Source: CAD feature listing. Evaluate the final solid. Frame: model axes, mm. A direction names the side the tool comes from. Coordinates: 2 decimals unless noted, no trailing zeros. Order: outer loops, then holes, each group sorted by start corner. A loop starts at its lowest first (then second) coordinate and runs counter-clockwise, first axis right, second up. Notation, with made-up numbers: (35, 88.25) - (56, 88.25) arc R18 ccw to (56, 106.25) - close; hole circle Ø4 at (23.25, 2). An arc over 180 degrees is marked (long way). One line per question, with ' | ' between items. Start each with the question number.
(1) Section B-B (y = 30.5). Return the cut outline in (x, z), then the cut area to 3 significant figures.
(2) Section C-C (y = 4). Return the cut outline in (x, z), then the cut area to 3 significant figures.
(3) Contact query for flat-ended pins moving along their axis: P1, Ø3, axis at x = 28, y = 22.44, coming from the +Z side; P2, Ø2, axis at x = 89.5, z = 0.5, coming from the +Y side. Output: stop coordinate, or through.
(4) Access query for faces 1 (the cylindrical face through (-9.54, 20, 0.03)), 2 (the flat face through (-42, 22, 0)). Directions: +Z, -Z, +X, -X, +Y, -Y. A direction counts if a zero-diameter tool reaches every point of the face in a straight line with its end or side. Return the directions, or none.
(5) Line query: line 1 along X through (y, z) = (14.5, 0.45); line 2 along Y through (x, z) = (28, -0.75); line 3 along X through (y, z) = (2, -1.7). Output: solid intervals per line, ascending.
(6) Draft query along Y for faces 3 (the flat face through (83, 12.443, 0)), 4 (the flat face through (27, 8, 2)), 5 (the cylindrical face through (103.154, 20.225, 0.028)), 6 (the cylindrical face through (67.31, 21.49, 0.03)). Return one class per face: +Y half, -Y half, draft (parallel to the pull), parting line (faces both ways), or undercut.
(7) Section D-D (z = 0.8). Count the separate pieces of the cut face and the enclosed holes in it, then the cut area to 3 significant figures.
(8) Section A-A (x = -46). Return the cut outline in (y, z).
from build123d import *

# Parameters (mm, degrees)
SKETCH1_W           = 156
SKETCH1_H           = 20
SKETCH1_W_2         = 8
BOSS_EXTRUDE1_DEPTH = 2
SKETCH2_R           = 2.5
CUT_EXTRUDE1_DEPTH  = 111.92580296
LPATTERN1_COUNT     = 5
LPATTERN1_PITCH     = 37
SKETCH3_R           = 3
CUT_EXTRUDE2_DEPTH  = 111.92580296


with BuildPart() as part:
    # Sketch1 → Boss-Extrude1 (new, symmetric)
    with BuildSketch(Plane.XY):
        with Locations((28, 2.442776735)):
            Rectangle(SKETCH1_W, SKETCH1_H)
        with Locations((102, 22.442776735)):
            Rectangle(SKETCH1_W_2, SKETCH1_H)
        with Locations((65, 22.442776735)):
            Rectangle(SKETCH1_W_2, SKETCH1_H)
        with Locations((28, 22.442776735)):
            Rectangle(SKETCH1_W_2, SKETCH1_H)
        with Locations((-9, 22.442776735)):
            Rectangle(SKETCH1_W_2, SKETCH1_H)
        with Locations((-46, 22.442776735)):
            Rectangle(SKETCH1_W_2, SKETCH1_H)
    extrude(amount=BOSS_EXTRUDE1_DEPTH, both=True)

    # Sketch2 → Cut-Extrude1 (cut, through all)
    with BuildSketch(Plane.XY.offset(2)):
        with Locations((-46, 22.442776735)):
            Circle(SKETCH2_R)
    cut_extrude1 = extrude(amount=-CUT_EXTRUDE1_DEPTH, mode=Mode.SUBTRACT)

    # LPattern1: Cut-Extrude1 ×5
    with Locations(*[(i * LPATTERN1_PITCH, 0, 0) for i in range(1, LPATTERN1_COUNT)]):
        add(cut_extrude1, mode=Mode.SUBTRACT)

    # Sketch3 → Cut-Extrude2 (cut, through all)
    with BuildSketch(Plane.XY.offset(2)):
        with Locations((28, 2.442776735)):
            Circle(SKETCH3_R)
        with Locations((96, 2.442776735)):
            Circle(SKETCH3_R)
        with Locations((-40, 2.442776735)):
            Circle(SKETCH3_R)
    extrude(amount=-CUT_EXTRUDE2_DEPTH, mode=Mode.SUBTRACT)


solid = part.part
Response values:
1) outline: (-50, -2) - (-42, -2) - (-42, 2) - (-50, 2) - close; (-13, -2) - (-5, -2) - (-5, 2) - (-13, 2) - close; (24, -2) - (32, -2) - (32, 2) - (24, 2) - close; (61, -2) - (69, -2) - (69, 2) - (61, 2) - close; (98, -2) - (106, -2) - (106, 2) - (98, 2) - close | area: 160 mm²
2) outline: (-50, -2) - (-42.56, -2) - (-42.56, 2) - (-50, 2) - close; (-37.44, -2) - (25.44, -2) - (25.44, 2) - (-37.44, 2) - close; (30.56, -2) - (93.44, -2) - (93.44, 2) - (30.56, 2) - close; (98.56, -2) - (106, -2) - (106, 2) - (98.56, 2) - close | area: 562 mm²
3) P1: passes through | P2: stops at y = 12.44
4) face 1: +Z, -Z | face 2: +Z, -Z, +Y
5) line 1: x = -50 to -42, -13 to -5, 24 to 32, 61 to 69, 98 to 106 | line 2: y = -7.56 to -0.56, 5.44 to 19.94, 24.94 to 32.44 | line 3: x = -50 to -42.97, -37.03 to 25.03, 30.97 to 93.03, 98.97 to 106
6) face 3: +Y half | face 4: draft | face 5: undercut | face 6: undercut
7) separate pieces: 1 | enclosed holes: 8 | area: 3,740 mm²
8) outline: (-7.56, -2) - (19.94, -2) - (19.94, 2) - (-7.56, 2) - close; (24.94, -2) - (32.44, -2) - (32.44, 2) - (24.94, 2) - close
